```python
from build123d import *

# Parameters (mm, degrees)
SKETCH_1_R          = 20
EXTRUDE_1_DEPTH     = 10
EXTRUDE_2_DEPTH     = 3
SKETCH_7_R          = 20
EXTRUDE_3_DEPTH     = 30
RIB_START           = -5
RIB_1_DEPTH         = 10
CUT_EXTRUDE_1_DEPTH = 92.515026089


# Read off the part's stored shape, not the designer's step: 筋1
with BuildPart() as part:
    # 草图1 → 凸台-拉伸1 (new body)
    with BuildSketch(Plane(origin=(0, 0, 0), x_dir=(1, 0, 0), z_dir=(0, 1, 0))):
        with BuildLine():
            Line((1.25, 19.960899278), (-78.4375, 24.951124098))
            ThreePointArc((-78.4375, 24.951124098), (-61.778275329, 17.116329922), (-55, 0))
            ThreePointArc((-55, 0), (-61.778275329, -17.116329922), (-78.4375, -24.951124098))
            Line((-78.4375, -24.951124098), (1.25, -19.960899278))
            ThreePointArc((1.25, -19.960899278), (-20, 0), (1.25, 19.960899278))
        make_face()
        with BuildLine():
            ThreePointArc((-55, 0), (-61.778275329, 17.116329922), (-78.4375, 24.951124098))
            Line((-78.4375, 24.951124098), (-78.4375, 14.918397828))
            ThreePointArc((-78.4375, 14.918397828), (-68.854653437, 10.038986503), (-65, 0))
            ThreePointArc((-65, 0), (-68.854653437, -10.038986503), (-78.4375, -14.918397828))
            Line((-78.4375, -14.918397828), (-78.4375, -24.951124098))
            ThreePointArc((-78.4375, -24.951124098), (-61.778275329, -17.116329922), (-55, 0))
        make_face()
        Circle(SKETCH_1_R)
    extrude(amount=EXTRUDE_1_DEPTH)

    # 草图5 → 凸台-拉伸2 (add)
    with BuildSketch(Plane(origin=(0, 10, 0), x_dir=(1, 0, 0), z_dir=(0, 1, 0))):
        with BuildLine():
            ThreePointArc((-78.4375, 24.951124098), (-55, 0), (-78.4375, -24.951124098))
            Line((-78.4375, -24.951124098), (-78.4375, -14.918397828))
            ThreePointArc((-78.4375, -14.918397828), (-65, 0), (-78.4375, 14.918397828))
            Line((-78.4375, 14.918397828), (-78.4375, 24.951124098))
        make_face()
    extrude(amount=EXTRUDE_2_DEPTH)

    # 草图7 → 凸台-拉伸3 (add)
    with BuildSketch(Plane(origin=(0, 10, 0), x_dir=(1, 0, 0), z_dir=(0, 1, 0))):
        with Locations(Location((0, 0, 0), (0, 0, 86.416678302))):
            Circle(SKETCH_7_R)
    extrude(amount=EXTRUDE_3_DEPTH)

    # 筋1 outline → 筋1 (add)
    with BuildSketch(Plane.XY.offset(RIB_START)):
        Polygon((-19.364916731, 30.34827147), (-51, 13), (-57, 13), (-57, 10), (-18, 10), (-18, 31.096774193), align=None)
    extrude(amount=RIB_1_DEPTH)

    # 草图9 → 切除-拉伸1 (cut, through all)
    with BuildSketch(Plane(origin=(0, 40, 0), x_dir=(1, 0, 0), z_dir=(0, 1, 0))):
        with BuildLine():
            Line((0, -5), (0, 5))
            Line((0, 5), (11.456439237, 5))
            ThreePointArc((11.456439237, 5), (-12.5, 0), (11.456439237, -5))
            Line((11.456439237, -5), (0, -5))
        make_face()
        with BuildLine():
            Line((11.456439237, 5), (0, 5))
            Line((0, 5), (0, -5))
            Line((0, -5), (11.456439237, -5))
            ThreePointArc((11.456439237, -5), (12.236328912, -2.553870546), (12.5, 0))
            ThreePointArc((12.5, 0), (12.236328912, 2.553870546), (11.456439237, 5))
        make_face()
        with BuildLine():
            Line((15, 5), (11.456439237, 5))
            ThreePointArc((11.456439237, 5), (12.236328912, 2.553870546), (12.5, 0))
            ThreePointArc((12.5, 0), (12.236328912, -2.553870546), (11.456439237, -5))
            Line((11.456439237, -5), (15, -5))
            Line((15, -5), (15, 5))
        make_face()
    extrude(amount=-CUT_EXTRUDE_1_DEPTH, mode=Mode.SUBTRACT)


solid = part.part
```
Model file for the job. Use its own axes, mm. A direction names the side the tool comes from. Coordinates: 2 decimals unless noted, no trailing zeros. Loops run counter-clockwise (first coordinate to the right, second up) from the corner with the lowest first, then second, coordinate; pieces in that order, holes last. Notation, with made-up numbers: M 42,21.5 L 95,21.5 A21 cw 95,26.5 Z; hole C 14.5,35.5 d6. An arc over 180 degrees is marked long. Use CSV: the item, a comma, the result in double quotes. Start each with the question number.
1. Probe probe 1 along Z at (x, y) = (0, 25); probe 2 along Y at (x, z) = (-35, 12.5); probe 3 along Y at (x, z) = (-59, 6). List the from-to ranges inside material, lowest first. Write a range as [from, to].
2. Tool access for faces 5 (the flat face through (15, 20, 0)), 6 (the flat face through (-39, 10, 15)), 7 (the flat face through (-39, 10, -15)): list every direction of +Z, -Z, +X, -X, +Y, -Y with a clear straight run to the whole face (end or side of a thin tool).
3. Band-saw the part on C-C, the plane x = -43. List the corners of the cut face in (y, z), then the cut area to 3 significant figures.
4. Flat gauge pins, fed straight in: pin 1 (2 mm diameter, centred on y = 8, z = -13, fed in from +X); pin 2 (3 mm diameter, centred on x = 13, y = 20.5, fed in from +Z); pin 3 (15 mm diameter, centred on x = 0, z = 0, fed in from +Y); pin 4 (1.5 mm diameter, centred on x = 8, y = 27, fed in from +Z). Where does each tip first touch, or does it go through?
5. Two-plate mould, pull along X, no slides. Class faces 1 (the flat face through (-41, 0, 0)), 2 (the flat face through (-34, 16, 5)), 3 (the cylindrical face through (-12.49, 20.28, -0.48)), 4 (the flat face through (-78.438, 6, -20)): pulls with the +X half, pulls with the -X half, needs draft (parallel to the pull), parting line crosses it, or undercut.
6. Band-saw the part on D-D, the plane y = 27. List the corners of the cut face in (x, z).
7. Band-saw the part on A-A, the plane y = 11.5. List the corners of the cut face in (x, z), then the cut area to 3 significant figures.
Entries:
1,probe 1,"z = [-20, -12.5], [12.5, 20]"
1,probe 2,"y = [0, 10]"
1,probe 3,"y = [0, 13]"
2,face 5,"+Y, -Y"
2,face 6,"+Z, +Y"
2,face 7,"-Z, +Y"
3,outline,"M 0,-22.73 L 10,-22.73 L 10,-5 L 17.39,-5 L 17.39,5 L 10,5 L 10,22.73 L 0,22.73 Z"
3,area,"529 mm2"
4,pin 1,"stops at x = 16"
4,pin 2,"stops at z = 16.36"
4,pin 3,"passes through"
4,pin 4,"stops at z = 18.64"
5,face 1,"needs draft"
5,face 2,"undercut"
5,face 3,"undercut"
5,face 4,"pulls with the -X half"
6,outline,"M -25.47,-5 L -19.36,-5 A20 ccw long -19.36,5 L -25.47,5 Z; hole M 11.46,-5 L 15,-5 L 15,5 L 11.46,5 A12.5 ccw long Z"
7,outline,"M -78.44,-24.95 A25 ccw -55.51,-5 L -19.36,-5 A20 ccw long -19.36,5 L -55.51,5 A25 ccw -78.44,24.95 L -78.44,14.92 A15 cw -78.44,-14.92 Z; hole M 11.46,-5 L 15,-5 L 15,5 L 11.46,5 A12.5 ccw long Z"
7,area,"1,690 mm2"
